from build123d import *

# Parameters (mm, degrees)
SKETCH1_R                       = 17.4
BOSS_EXTRUDE1_DEPTH             = 15.4
SKETCH2_R                       = 18
BOSS_EXTRUDE2_DEPTH             = 30.7
SKETCH3_R                       = 18.4
BOSS_EXTRUDE3_DEPTH             = 26.5
SKETCH4_R                       = 6
BOSS_EXTRUDE4_DEPTH             = 6.5
SKETCH5_R                       = 3
BOSS_EXTRUDE5_DEPTH             = 15.5
CUT_EXTRUDE1_DEPTH              = 13
TAP_DRILL_FOR_M3X0_5_TAP1_D     = 2.5
TAP_DRILL_FOR_M3X0_5_TAP1_DEPTH = 10.76


with BuildPart() as part:
    # Sketch1 → Boss-Extrude1 (new body)
    with BuildSketch(Plane.XY):
        Circle(SKETCH1_R)
    extrude(amount=BOSS_EXTRUDE1_DEPTH)

    # Sketch2 → Boss-Extrude2 (add)
    with BuildSketch(Plane.XY.offset(15.4)):
        Circle(SKETCH2_R)
    extrude(amount=BOSS_EXTRUDE2_DEPTH)

    # Sketch3 → Boss-Extrude3 (add)
    with BuildSketch(Plane.XY.offset(46.1)):
        Circle(SKETCH3_R)
    extrude(amount=BOSS_EXTRUDE3_DEPTH)

    # Sketch4 → Boss-Extrude4 (add)
    with BuildSketch(Plane.XY.offset(72.6)):
        with Locations((0, -7)):
            Circle(SKETCH4_R)
    extrude(amount=BOSS_EXTRUDE4_DEPTH)

    # Sketch5 → Boss-Extrude5 (add)
    with BuildSketch(Plane.XY.offset(79.1)):
        with Locations((0, -7)):
            Circle(SKETCH5_R)
    extrude(amount=BOSS_EXTRUDE5_DEPTH)

    # Sketch6 → Cut-Extrude1 (cut)
    with BuildSketch(Plane.XY.offset(94.6)):
        with BuildLine():
            Line((-1.8, -4.6), (1.8, -4.6))
            ThreePointArc((1.8, -4.6), (0, -4), (-1.8, -4.6))
        make_face()
    extrude(amount=-CUT_EXTRUDE1_DEPTH, mode=Mode.SUBTRACT)

    # Tap Drill for M3x0.5 Tap1
    with Locations(Plane.XY.offset(72.6)):
        with Locations((-15.5, 0), (-7.75, 13.423393759), (7.75, 13.423393759), (15.5, 0), (7.75, -13.423393759), (-7.75, -13.423393759)):
            Hole(TAP_DRILL_FOR_M3X0_5_TAP1_D / 2, depth=TAP_DRILL_FOR_M3X0_5_TAP1_DEPTH)


solid = part.part
Could you check a few things on this model? Use its own coordinates, in mm. A direction names the side the tool comes from. Coordinates: 2 decimals unless noted, no trailing zeros. Write each loop counter-clockwise with the first axis right and the second up, starting at its lowest first coordinate (ties: lowest second). Pieces come first, ordered by that corner, then holes. Notation, with made-up numbers: M -17.75,-21 L 9.25,-21 A18 ccw 9.25,1 Z; hole C 67.25,-5.5 d3. An arc over 180 degrees is marked long. One line per question, with ' | ' between items.
1) If we mould it in two halves opening along Y, with no side actions, what happens to faces 1 (the face through (8.67, -12.58, 67.14)), 2 (the face through (-3, -8, 79.1)), 3 (the face through (-14.25, 0.05, 67.14)), 4 (the face through (-2.343, 17.847, 30.535))? For each: released by +Y, released by -Y, zero draft, split by the parting line, or undercut.
Checks:
face 1: undercut | face 2: zero draft | face 3: undercut | face 4: split by the parting line
2) I need wall thicknesses on probe 1 along Y at (x, z) = (-7.75, 64.5); probe 2 along Y at (x, z) = (8, 64); probe 3 along Z at (x, y) = (0, 16.5). Which ranges of each line are inside material? Lowest first, please. Write a range as [from, to].
Checks:
probe 1: [-16.69, -14.67], [-12.17, 12.17], [14.67, 16.69] | probe 2: [-16.57, -14.65], [-12.2, 12.2], [14.65, 16.57] | probe 3: [0, 72.6]
3) For pin 1 Ø1 at (y, z) = (-2, 63) entering from -X; pin 2 Ø1 at (x, y) = (7.5, 5.5) entering from +Z; pin 3 Ø0.5 at (x, y) = (0, -4) entering from +Z, each with a flat end and sliding along its axis, tell me the tip position at first contact or that it passes through.
Checks:
pin 1: x = -18.34 | pin 2: z = 72.6 | pin 3: z = 81.6
4) Imagine slicing it at C-C, the plane z = 60.5. Write out the boundary of the cut face in (x, y), and give its area (3 significant figures).
Checks:
outline: C 0,0 d36.8 | area: 1,060 mm²
5) Imagine slicing it at A-A, the plane x = 0. Write out the boundary of the cut face in (y, z), and give its area (3 significant figures).
Checks:
outline: M -18.4,46.1 L -18,46.1 L -18,15.4 L -17.4,15.4 L -17.4,0 L 17.4,0 L 17.4,15.4 L 18,15.4 L 18,46.1 L 18.4,46.1 L 18.4,72.6 L -1,72.6 L -1,79.1 L -4,79.1 L -4,81.6 L -4.6,81.6 L -4.6,94.6 L -10,94.6 L -10,79.1 L -13,79.1 L -13,72.6 L -18.4,72.6 Z | area: 2,780 mm²
6) Imagine slicing it at D-D, the plane y = -8. Write out the boundary of the cut face in (x, z).
Checks:
outline: M -16.57,46.1 L -16.12,46.1 L -16.12,15.4 L -15.45,15.4 L -15.45,0 L 15.45,0 L 15.45,15.4 L 16.12,15.4 L 16.12,46.1 L 16.57,46.1 L 16.57,72.6 L 5.92,72.6 L 5.92,79.1 L 2.83,79.1 L 2.83,94.6 L -2.83,94.6 L -2.83,79.1 L -5.92,79.1 L -5.92,72.6 L -16.57,72.6 Z
7) Imagine slicing it at B-B, the plane y = 0. Write out the boundary of the cut face in (x, z), and give its area (3 significant figures).
Checks:
outline: M -18.4,46.1 L -18,46.1 L -18,15.4 L -17.4,15.4 L -17.4,0 L 17.4,0 L 17.4,15.4 L 18,15.4 L 18,46.1 L 18.4,46.1 L 18.4,72.6 L 16.75,72.6 L 16.75,61.84 L 14.25,61.84 L 14.25,72.6 L -14.25,72.6 L -14.25,61.84 L -16.75,61.84 L -16.75,72.6 L -18.4,72.6 Z | area: 2,560 mm²
8) For faces 5 (the face through (-6, -7, 76)), 6 (the face through (-3.772, -16.986, 7.592)), 7 (the face through (0, -4.6, 88)), which set-ups out of +Z, -Z, +X, -X, +Y, -Y let a thin tool reach every point of the face, with its end or its side?
Checks:
face 5: +Z | face 6: -Z | face 7: +Z, +X, -X, +Y
